Verification items for the finished model (mm, model axes). Face numbers are marked on the shaded views. A direction names the side the tool comes from. Give positions to 0.01 mm unless a question says otherwise; leave off trailing zeros. Order: outer loops, then holes, each group sorted by start corner. A loop starts at its lowest first (then second) coordinate and runs counter-clockwise, first axis right, second up. Notation, with made-up numbers: (-0.75, 13) -> (32.25, 13) arc R20 cw to (32.25, 23) -> close; hole circle Ø8 at (75.25, 44.25). An arc over 180 degrees is marked (long way). One line per question, with ' | ' between items. Start each with the question number.
Q1. Mould release check, pull along X, two halves, no side actions. Record for the marked faces 1, 2, 3 and 4: released by +X, released by -X, zero draft, split by the parting line, or undercut.
Q2. Material ranges on probe 1 along X at (y, z) = (18.25, -14.75) (3 decimals); probe 2 along Z at (x, y) = (15.75, 5); probe 3 along Z at (x, y) = (21.5, 16.5), recorded low to high. Write a range as [from, to].
Q3. Section check A-A on z = -20.75. Record the cut outline in (x, y), plus the area to 3 significant figures.
Q4. Access from +Z, -Z, +X, -X, +Y, -Y to the whole of each face (thin tool, end or side, straight path). Record for the marked faces 5, 6 and 7.
Q5. Go/stop test with flat-tipped pins: pin 1 (4 mm diameter, centred on x = 20.5, y = 13, fed in from +Z); pin 2 (2 mm diameter, centred on x = 12.5, z = -6.5, fed in from -Y). Record where each tip stops, or that it passes through.
Q6. Section check B-B on x = 22.5. Record the cut outline in (y, z), plus the area to 3 significant figures.
Q7. Section check D-D on z = -10.5. Record the cut outline in (x, y) (3 decimals), plus the area to 3 significant figures.
from build123d import *

# Parameters (mm, degrees)
SKETCH1_W           = 27
SKETCH1_H           = 32
BOSS_EXTRUDE1_DEPTH = 31.58
SKETCH3_W           = 20
SKETCH3_H           = 23
CUT_EXTRUDE1_DEPTH  = 30
SKETCH4_W           = 7.5
SKETCH4_H           = 3.655478676
CUT_EXTRUDE2_DEPTH  = 25
SKETCH5_R           = 6.5
SKETCH5_R_2         = 1.269841787
CUT_EXTRUDE4_DEPTH  = 10
SKETCH6_W           = 27
SKETCH6_H           = 3.072558681
CUT_EXTRUDE5_DEPTH  = 32.58
FILLET2_R           = 5
SKETCH7_R           = 2.55
BOSS_EXTRUDE2_DEPTH = 2.83
SKETCH8_W           = 3.381092642
SKETCH8_H           = 7.1
SKETCH8_H_2         = 11.3
SKETCH8_W_2         = 3.125
BOSS_EXTRUDE4_DEPTH = 30
SKETCH11_W          = 2.605806733
SKETCH11_H          = 28.316955939
CUT_EXTRUDE10_DEPTH = 32.58
SKETCH12_W          = 21.788386534
SKETCH12_H          = 2.319503847
CUT_EXTRUDE11_DEPTH = 32.58
SKETCH13_W          = 21.788386534
SKETCH13_H          = 2.858824784
CUT_EXTRUDE12_DEPTH = 30.437937473
CUT_EXTRUDE13_DEPTH = 10
SKETCH15_R          = 1
CUT_EXTRUDE14_DEPTH = 3


with BuildPart() as part:
    # Sketch1 → Boss-Extrude1 (new body)
    with BuildSketch(Plane(origin=(0, 0, 0), x_dir=(1, 0, 0), z_dir=(0, 1, 0))):
        with Locations((13.5, 16)):
            Rectangle(SKETCH1_W, SKETCH1_H)
    extrude(amount=BOSS_EXTRUDE1_DEPTH)

    # Sketch3 → Cut-Extrude1 (cut)
    with BuildSketch(Plane(origin=(0, 31.58, 0), x_dir=(1, 0, 0), z_dir=(0, 1, 0))):
        with Locations((13.5, 16.844521324)):
            Rectangle(SKETCH3_W, SKETCH3_H)
    extrude(amount=-CUT_EXTRUDE1_DEPTH, mode=Mode.SUBTRACT)

    # Sketch4 → Cut-Extrude2 (cut)
    with BuildSketch(Plane(origin=(0, 31.58, 0), x_dir=(1, 0, 0), z_dir=(0, 1, 0))):
        with Locations((13.5, 30.172260662)):
            Rectangle(SKETCH4_W, SKETCH4_H)
    extrude(amount=-CUT_EXTRUDE2_DEPTH, mode=Mode.SUBTRACT)

    # Sketch5 → Cut-Extrude4 (cut)
    with BuildSketch(Plane(origin=(0, 0, -32), x_dir=(-1, 0, 0), z_dir=(0, 0, -1))):
        with Locations((-13.618907358, 13.887482267)):
            Circle(SKETCH5_R)
        with Locations((-13.618907358, 13.887482267)):
            Circle(SKETCH5_R_2, mode=Mode.SUBTRACT)
    extrude(amount=-CUT_EXTRUDE4_DEPTH, mode=Mode.SUBTRACT)

    # Sketch6 → Cut-Extrude5 (cut, through all)
    with BuildSketch(Plane(origin=(0, 31.58, 0), x_dir=(1, 0, 0), z_dir=(0, 1, 0))):
        with Locations((13.5, 1.536279341)):
            Rectangle(SKETCH6_W, SKETCH6_H)
    extrude(amount=-CUT_EXTRUDE5_DEPTH, mode=Mode.SUBTRACT)

    # Fillet2
    fillet2_edges = [part.edges().sort_by_distance(p)[0] for p in [
        (13.5, 0, -32),
        (0, 0, -17.53627934),
        (27, 0, -17.53627934),
        (13.5, 0, -3.072558681),
        (0, 15.79, -3.072558681),
        (27, 15.79, -3.072558681),
        (0, 15.79, -32),
        (27, 15.79, -32),
    ]]
    fillet(fillet2_edges, radius=FILLET2_R)

    # Sketch7 → Boss-Extrude2 (add)
    with BuildSketch(Plane.XY.offset(-3.072558681)):
        with Locations((13.618907358, 12.657)):
            Circle(SKETCH7_R)
    extrude(amount=BOSS_EXTRUDE2_DEPTH)

    # Sketch8 → Boss-Extrude4 (add)
    with BuildSketch(Plane(origin=(0, 31.58, 0), x_dir=(1, 0, 0), z_dir=(0, 1, 0))):
        with Locations((21.809453679, 24.794521324)):
            Rectangle(SKETCH8_W, SKETCH8_H)
        with Locations((21.809453679, 10.994521324)):
            Rectangle(SKETCH8_W, SKETCH8_H_2)
        with Locations((5.0625, 24.794521324)):
            Rectangle(SKETCH8_W_2, SKETCH8_H)
        with Locations((5.0625, 10.994521324)):
            Rectangle(SKETCH8_W_2, SKETCH8_H_2)
    extrude(amount=-BOSS_EXTRUDE4_DEPTH)

    # Sketch11 → Cut-Extrude10 (cut, through all)
    with BuildSketch(Plane(origin=(0, 31.58, 0), x_dir=(1, 0, 0), z_dir=(0, 1, 0))):
        with Locations((1.302903367, 17.841522031)):
            Rectangle(SKETCH11_W, SKETCH11_H)
        Polygon((24.394193267, 18.51018278), (24.394193267, 32), (27, 32), (27, 2.645827608), (24.394193267, 2.645827608), (24.394193267, 18.158757191), align=None)
    extrude(amount=-CUT_EXTRUDE10_DEPTH, mode=Mode.SUBTRACT)

    # Sketch12 → Cut-Extrude11 (cut, through all)
    with BuildSketch(Plane(origin=(0, 31.58, 0), x_dir=(1, 0, 0), z_dir=(0, 1, 0))):
        with Locations((13.5, 30.840248077)):
            Rectangle(SKETCH12_W, SKETCH12_H)
    extrude(amount=-CUT_EXTRUDE11_DEPTH, mode=Mode.SUBTRACT)

    # Sketch13 → Cut-Extrude12 (cut, through all)
    with BuildSketch(Plane(origin=(0, 0, -29.680496153), x_dir=(-1, 0, 0), z_dir=(0, 0, -1))):
        with Locations((-13.5, 1.429412392)):
            Rectangle(SKETCH13_W, SKETCH13_H)
    extrude(amount=-CUT_EXTRUDE12_DEPTH, mode=Mode.SUBTRACT)

    # Sketch14 → Cut-Extrude13 (cut)
    with BuildSketch(Plane(origin=(0, 0, -29.680496153), x_dir=(-1, 0, 0), z_dir=(0, 0, -1))):
        Polygon((-20.118907358, 13.887482267), (-20.118907358, 31.58), (-7.265621144, 31.58), (-7.118907358, 13.887482267), align=None)
    extrude(amount=-CUT_EXTRUDE13_DEPTH, mode=Mode.SUBTRACT)

    # Sketch15 → Cut-Extrude14 (cut)
    with BuildSketch(Plane(origin=(0, 31.58, 0), x_dir=(1, 0, 0), z_dir=(0, 1, 0))):
        with Locations((4.525, 26.375422159)):
            Circle(SKETCH15_R)
        with Locations((22.218907358, 26.375422159)):
            Circle(SKETCH15_R)
    extrude(amount=-CUT_EXTRUDE14_DEPTH, mode=Mode.SUBTRACT)


solid = part.part
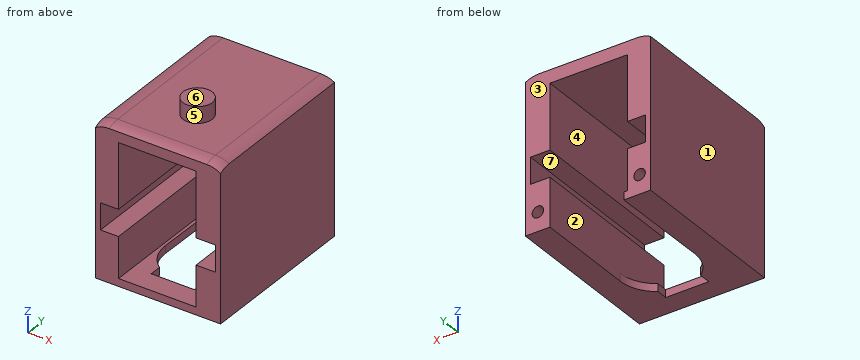
Filled in:
1) face 1: released by -X | face 2: undercut | face 3: zero draft | face 4: undercut
2) probe 1: [2.606, 6.625], [20.119, 24.394] | probe 2: [-29.68, -28.34], [-5.34, -3.07] | probe 3: [-29.68, -21.24], [-16.64, -3.07]
3) outline: (2.61, 2.86) -> (3.5, 2.86) -> (3.5, 31.58) -> (2.61, 31.58) -> close; (23.5, 2.86) -> (24.39, 2.86) -> (24.39, 31.58) -> (23.5, 31.58) -> close | area: 51.4 mm²
4) face 5: +Z | face 6: +Z, +X, -X, +Y, -Y | face 7: +Y, -Y
5) pin 1: z = -3.07 | pin 2: through
6) outline: (2.86, -29.68) -> (31.58, -29.68) -> (31.58, -27.34) -> (28.58, -27.34) -> (28.58, -25.42) -> (31.58, -25.42) -> (31.58, -21.24) -> (2.86, -21.24) -> close; (2.86, -16.64) -> (31.58, -16.64) -> (31.58, -3.1) -> (5, -3.1) arc R4.97 ccw to (2.86, -3.58) -> close | area: 625 mm²
7) outline: (2.606, 2.859) -> (6.625, 2.859) -> (6.625, 31.58) -> (2.606, 31.58) -> close; (20.119, 2.859) -> (24.394, 2.859) -> (24.394, 31.58) -> (20.119, 31.58) -> close | area: 238 mm²
